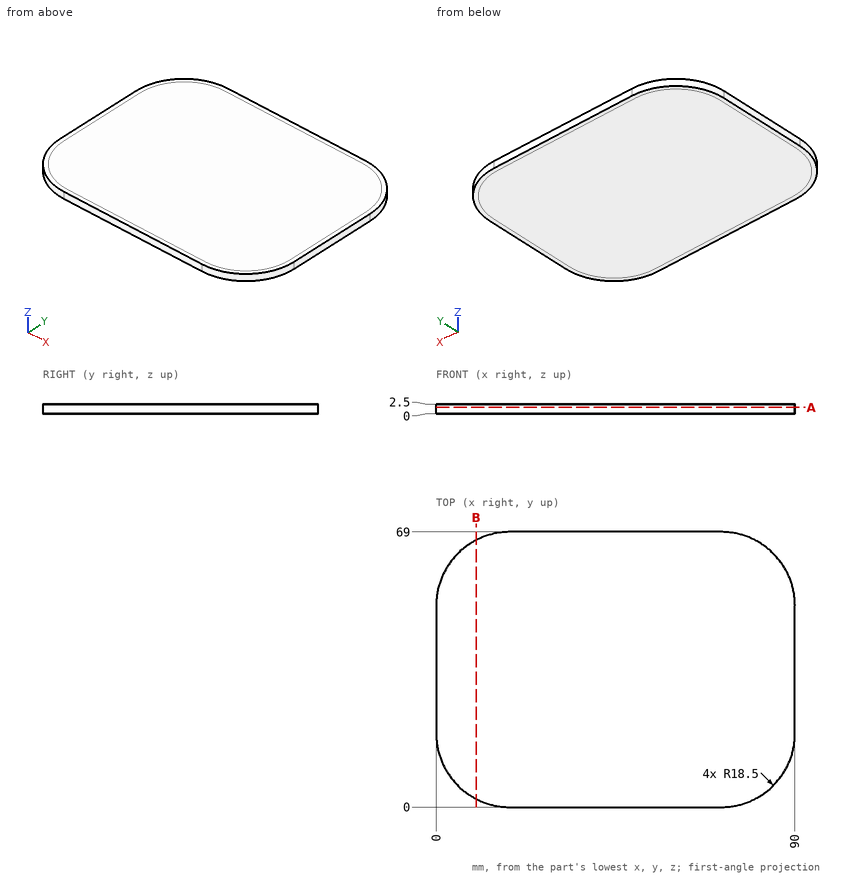
Job drawing, mm, ordinate dimensions from the low corner. One solid piece. Give positions to 0.01 mm unless a question says otherwise; leave off trailing zeros. Loops run counter-clockwise (first coordinate to the right, second up) from the corner with the lowest first, then second, coordinate; pieces in that order, holes last. Notation, with made-up numbers: (87.25, 32) - (113.25, 32) arc R21 ccw to (113.25, 44) - close; hole circle Ø4 at (89, 11.25). An arc over 180 degrees is marked (long way). Use one line per item in the form item = value.
(1) Drill centre lines: L1, parallel to X at y = 17, z = 1.8; L2, parallel to Y at x = 75, z = 1.4; L3, parallel to X at y = 62, z = 1.7. Where is each one in solid material? Low to high.
Determined:
L1 = 0.06 to 89.94
L2 = 0.33 to 68.67
L3 = 4.01 to 85.99
(2) Cut at A-A (z = 1.65). Give the cut face in (x, y).
Determined:
outline = (0, 18.5) arc R18.5 ccw to (18.5, 0) - (71.5, 0) arc R18.5 ccw to (90, 18.5) - (90, 50.5) arc R18.5 ccw to (71.5, 69) - (18.5, 69) arc R18.5 ccw to (0, 50.5) - close
(3) Cut at B-B (x = 10). Give the cut face in (y, z).
Determined:
outline = (2.07, 0) - (66.93, 0) - (66.93, 2.5) - (2.07, 2.5) - close
